The model under review builds one solid part; all positions refer to its coordinate system, in mm. Face numbers are marked on the shaded views. Coordinates: 2 decimals unless noted, no trailing zeros. Order: outer loops, then holes, each group sorted by start corner. A loop starts at its lowest first (then second) coordinate and runs counter-clockwise, first axis right, second up.
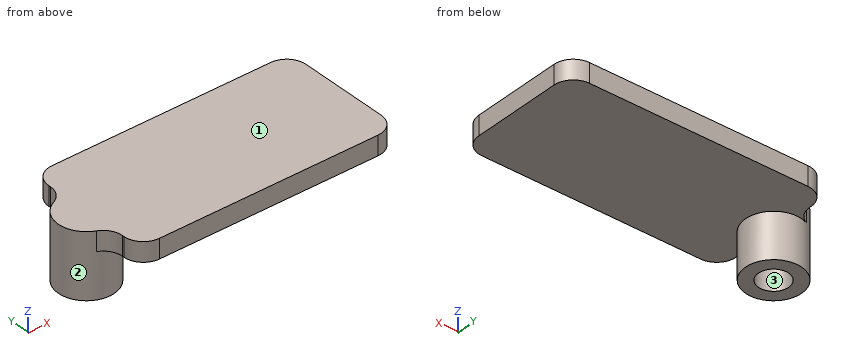
Autodesk Inventor part; units mm, degrees
ref_plane "YZ Plane" through (0, 0, 0) normal (1, 0, 0) x (0, 1, 0)
ref_plane "XZ Plane" through (0, 0, 0) normal (0, 1, 0) x (-1, 0, 0)
ref_plane "XY Plane" through (0, 0, 0) normal (0, 0, 1) x (1, 0, 0)
sketch "Sketch3" plane through (0, 0, 0) normal (0, 0, 1) x (1, 0, 0)
  circle A0 centre (0, 0) radius 2.35
  circle A1 centre (0, 0) radius 4.35
  dimension "d8" = 4.7
  dimension "d9" = 2
extrude "Extrusion3" add sketch "Sketch3" against normal blind 10
sketch "Sketch4" plane through (0, 0, 0) normal (0, 0, 1) x (1, 0, 0)
  circle A0 centre (0, 0) radius 4.35
  circle A1 centre (0, 0) radius 2.35
  line L0 (0, 0) -> (40, 0)
  line L1 (40, 0) -> (40, 10)
  line L2 (40, 10) -> (0, 10)
  line L3 (0, 10) -> (0, 0)
  line L4 (40, 0) -> (40, -10)
  line L5 (40, -10) -> (0, -10)
  line L6 (0, -10) -> (0, 0)
  point P0 (0, 4.35)
  point P1 (0, -4.35)
  dimension "d12" = 40
  dimension "d13" = 10
extrude "Extrusion4" add sketch "Sketch4" against normal blind 3 contours L0 L4 L5 L6 A0 | A0 L3 L2 L1 L0
fillet "Fillet1" radius 3 6 edges at (0, -4.35, -1.5) (0, 4.35, -1.5) (0, -10, -1.5) (0, 10, -1.5) (40, 10, -1.5) (40, -10, -1.5)
sketch "Sketch5" plane through (0, 0, 0) normal (0, 0, 1) x (1, 0, 0)
  circle A0 centre (0, 0) radius 2.35
extrude "Extrusion5" add sketch "Sketch5" against normal blind 6.5
sketch "Sketch6" plane through (0, 0, -3) normal (0, 0, -1) x (-1, 0, 0)
  arc A0 (-40, -7) -> (-37, -10) centre (-37, -7) ccw
  line L0 (-37, -10) -> (-3, -10)
  arc A1 (-3, -10) -> (0, -7) centre (-3, -7) ccw
  line L1 (0, -7) -> (0, -6.7099)
  arc A2 (1.7755, -3.9712) -> (0, -6.7099) centre (3, -6.7099) ccw
  arc A3 (1.7755, 3.9712) -> (1.7755, -3.9712) centre (0, 0) ccw
  arc A4 (0, 6.7099) -> (1.7755, 3.9712) centre (3, 6.7099) ccw
  line L2 (0, 6.7099) -> (0, 7)
  arc A5 (0, 7) -> (-3, 10) centre (-3, 7) ccw
  line L3 (-3, 10) -> (-37, 10)
  arc A6 (-37, 10) -> (-40, 7) centre (-37, 7) ccw
  line L4 (-40, 7) -> (-40, -7)
  line L5 (-20, -10) -> (-20, 10)
  line L6 (-40, 0) -> (-20, 0)
  circle A7 centre (-30, 0) radius 5.279
  dimension "d19" = 10.558
properties part number "TutupTank"
(1) For pin 1 Ø1 at (x, y) = (16.5, 1) entering from -Z; pin 2 Ø6 at (y, z) = (5, -8.5) entering from -X; pin 3 Ø6 at (y, z) = (6.5, -6) entering from -X, all flat-tipped, find the tip position at first contact; note any pin that passes through.
A:
pin 1: stops at z = -3
pin 2: stops at x = -3.86
pin 3: stops at x = -2.58
(2) Wall thickness on probe 1 along Y at (x, z) = (0, -8.6); probe 2 along Z at (x, y) = (12, 5); probe 3 along X at (y, z) = (1, -7.75): over which ranges is each line inside the solid? List them lowest first.
A:
probe 1: y = -4.35 to -2.35, 2.35 to 4.35
probe 2: z = -3 to 0
probe 3: x = -4.23 to -2.13, 2.13 to 4.23
(3) We need section A-A, the plane y = 0. Write out the cut boundary in (x, z), and give its area (4 significant figures).
A:
outline: (-4.35, -10) - (-2.35, -10) - (-2.35, -6.5) - (2.35, -6.5) - (2.35, -10) - (4.35, -10) - (4.35, -3) - (40, -3) - (40, 0) - (-4.35, 0) - close
area: 177.5 mm2
(4) Draft analysis for pull direction X (two halves, no side actions). For the marked faces 1, 2 and 3, state which applies: released by +X, released by -X, zero draft, split by the parting line, or undercut.
A:
face 1: zero draft
face 2: split by the parting line
face 3: undercut
(5) We need section D-D, the plane x = 9. Write out the cut boundary in (y, z).
A:
outline: (-10, -3) - (10, -3) - (10, 0) - (-10, 0) - close
(6) We need section B-B, the plane z = -1.5. Write out the cut boundary in (x, y), and give its area (3 significant figures).
A:
outline: (-1.78, -3.97) arc R3 cw to (0, -6.71) - (0, -7) arc R3 ccw to (3, -10) - (37, -10) arc R3 ccw to (40, -7) - (40, 7) arc R3 ccw to (37, 10) - (3, 10) arc R3 ccw to (0, 7) - (0, 6.71) arc R3 cw to (-1.78, 3.97) arc R4.35 ccw to start
area: 824 mm2
(7) We need section C-C, the plane z = -8.5. Write out the cut boundary in (x, y).
A:
outline: circle Ø8.7 at (0, 0); hole circle Ø4.7 at (0, 0)
